from build123d import *

# Parameters (mm, degrees)
SKETCH1_W           = 152.4
SKETCH1_H           = 114.3
BOSS_EXTRUDE1_DEPTH = 3.175
SKETCH2_W           = 152.4
SKETCH2_H           = 3.175
BOSS_EXTRUDE2_DEPTH = 406.4
FILLET1_R           = 2.54
FILLET2_R           = 5.08
SKETCH3_R           = 30.988
SKETCH3_R_2         = 2.54
SKETCH3_R_3         = 2.159
SKETCH3_R_4         = 2.15
CUT_EXTRUDE1_DEPTH  = 418.41289211


with BuildPart() as part:
    # Sketch1 → Boss-Extrude1 (new body)
    with BuildSketch(Plane(origin=(0, 0, 0), x_dir=(1, 0, 0), z_dir=(0, 1, 0))):
        Rectangle(SKETCH1_W, SKETCH1_H)
    extrude(amount=BOSS_EXTRUDE1_DEPTH)

    # Sketch2 → Boss-Extrude2 (add)
    with BuildSketch(Plane(origin=(0, 3.175, 0), x_dir=(1, 0, 0), z_dir=(0, 1, 0))):
        with Locations((0, -55.5625)):
            Rectangle(SKETCH2_W, SKETCH2_H)
    extrude(amount=BOSS_EXTRUDE2_DEPTH)

    # Fillet1
    fillet1_edges = [part.edges().sort_by_distance(p)[0] for p in [
        (0, 3.175, 53.975),
        (0, 0, 57.15),
    ]]
    fillet(fillet1_edges, radius=FILLET1_R)

    # Fillet2
    fillet2_edges = [part.edges().sort_by_distance(p)[0] for p in [
        (-76.2, 409.575, 55.5625),
        (76.2, 409.575, 55.5625),
        (-76.2, 1.5875, -57.15),
        (76.2, 1.5875, -57.15),
    ]]
    fillet(fillet2_edges, radius=FILLET2_R)

    # Sketch3 → Cut-Extrude1 (cut, through all)
    with BuildSketch(Plane(origin=(0, 3.175, 0), x_dir=(1, 0, 0), z_dir=(0, 1, 0))):
        with Locations(Location((-25.4, 3.81, 0), (0, 0, 270))):
            Circle(SKETCH3_R)
        with Locations(Location((15.875, 44.958, 0), (0, 0, 270))):
            Circle(SKETCH3_R_2)
        with Locations(Location((-66.675, -37.465, 0), (0, 0, 270))):
            Circle(SKETCH3_R_2)
        with Locations(Location((15.875, -37.465, 0), (0, 0, 270))):
            Circle(SKETCH3_R_2)
        with Locations(Location((30.988, 44.45, 0), (0, 0, 270))):
            Circle(SKETCH3_R_3)
        with Locations(Location((60.93860251, 44.46, 0), (0, 0, 270))):
            Circle(SKETCH3_R_4)
        with Locations(Location((60.96, 14.478, 0), (0, 0, 270))):
            Circle(SKETCH3_R_3)
        with Locations(Location((30.93860251, 14.478, 0), (0, 0, 270))):
            Circle(SKETCH3_R_3)
        with Locations(Location((-66.675, 45.085, 0), (0, 0, 270))):
            Circle(SKETCH3_R_2)
    extrude(amount=-CUT_EXTRUDE1_DEPTH, mode=Mode.SUBTRACT)


solid = part.part
Geometry: final body of the model. Coordinates: model frame, mm. A direction names the side the tool comes from. Give positions to 0.01 mm unless a question says otherwise; leave off trailing zeros. Write each loop counter-clockwise with the first axis right and the second up, starting at its lowest first coordinate (ties: lowest second). Pieces come first, ordered by that corner, then holes. Notation, with made-up numbers: (-9, -18.75) - (-2, -18.75) arc R8 cw to (-2, -5.75) - close; hole circle Ø6 at (-19, 79). An arc over 180 degrees is marked (long way). Return JSON: item names as keys, results as strings. Group by question number.
1) First-contact query: P1, Ø1, axis at x = -13, z = -32.5, coming from the +Y side (3 decimals); P2, Ø3, axis at x = -66.675, z = 37.465, coming from the -Y side; P3, Ø12, axis at x = 37, y = 342.5, coming from the -Z side (3 decimals). Flat tips, straight axial feed; report the tip coordinate or a pass-through.
2) Mould query, pull axis X, two halves, no side actions, for faces 3 (the flat face through (-76.2, 201, 55)), 4 (the flat face through (-1, 203, 57.15)), 5 (the cylindrical face through (-55.65, 1.61, -10.53)). Classes: released by +X, released by -X, zero draft, split by the parting line, or undercut.
3) Section B-B on z = -3.81. Return the cut outline in (x, y) (3 decimals), plus the area to 3 significant figures.
4) Section C-C on z = 12. Return the cut outline in (x, y) (3 decimals), plus the area to 3 significant figures.
5) Section D-D on y = 320.5. Return the cut outline in (x, z) (3 decimals).
6) Set-up query: faces 1 (the flat face through (76.2, 201, 55)), 2 (the flat face through (16, 3.175, -4)). Return all of +Z, -Z, +X, -X, +Y, -Y with unobstructed straight access to the full face (end or side cutting, diameter ignored); none if empty.
7) Line query: line 1 (X direction, y = 2, z = -44.45); line 2 (Z direction, x = -16.5, y = 73) (3 decimals); line 3 (Y direction, x = -22.5, z = 32.5) (3 decimals). Output: solid intervals per line, ascending.
8) Section A-A on x = -25.4. Return the cut outline in (y, z) (3 decimals).
Filled in:
{
 "1": {"P1": "stops at y = 3.175", "P2": "passes through", "P3": "stops at z = 53.975"},
 "2": {"face 3": "released by -X", "face 4": "zero draft", "face 5": "undercut"},
 "3": {"outline": "(-76.2, 0) - (-56.388, 0) - (-56.388, 3.175) - (-76.2, 3.175) - close; (5.588, 0) - (76.2, 0) - (76.2, 3.175) - (5.588, 3.175) - close", "area": "287 mm^2"},
 "4": {"outline": "(-76.2, 0) - (-52.051, 0) - (-52.051, 3.175) - (-76.2, 3.175) - close; (1.251, 0) - (76.2, 0) - (76.2, 3.175) - (1.251, 3.175) - close", "area": "315 mm^2"},
 "5": {"outline": "(-76.2, 53.975) - (76.2, 53.975) - (76.2, 57.15) - (-76.2, 57.15) - close"},
 "6": {"face 1": "+Z, -Z, +X, +Y, -Y", "face 2": "-Z, +X, -X, +Y"},
 "7": {"line 1": "x = -76.2 to -69.13, -64.22 to 13.39, 18.36 to 28.83, 33.15 to 58.79, 63.09 to 76.2", "line 2": "z = 53.975 to 57.15", "line 3": "y = 0 to 3.175"},
 "8": {"outline": "(0, -57.15) - (3.175, -57.15) - (3.175, -34.798) - (0, -34.798) - close; (0, 27.178) - (3.175, 27.178) - (3.175, 51.435) arc R2.54 cw to (5.715, 53.975) - (409.575, 53.975) - (409.575, 57.15) - (2.54, 57.15) arc R2.54 ccw to (0, 54.61) - close"}
}
